```python
from build123d import *

# Parameters (mm, degrees)
SKETCH010_W     = 10
SKETCH010_H     = 20
PAD004_DEPTH    = 1.2
SKETCH011_R     = 0.7
POCKET004_DEPTH = 1.201
SKETCH012_W     = 10
SKETCH012_H     = 20
PAD005_DEPTH    = 0.2
SKETCH014_W     = 10
SKETCH014_H     = 20
PAD006_DEPTH    = 2
POCKET005_DEPTH = 2
SKETCH015_W     = 10
SKETCH015_H     = 20
PAD007_DEPTH    = 2.5
SKETCH016_R     = 2.2
SKETCH016_W     = 5.8
SKETCH016_H     = 2.7
SKETCH016_W_2   = 2.5
SKETCH016_H_2   = 10.776226
POCKET006_DEPTH = 2.5
FILLET_R        = 3


with BuildPart() as part:
    # Sketch010 → Pad004 (new body)
    with BuildSketch(Plane.XY):
        Rectangle(SKETCH010_W, SKETCH010_H)
    extrude(amount=PAD004_DEPTH)

    # Sketch011 → Pocket004 (cut, through all)
    with BuildSketch(Plane.XY.offset(1.2)):
        with Locations((-1.27, -6.75)):
            Circle(SKETCH011_R)
        with Locations((1.27, -6.75)):
            Circle(SKETCH011_R)
        with Locations((-2, 7.25)):
            Circle(SKETCH011_R)
        with Locations((-2, -1.75)):
            Circle(SKETCH011_R)
        with Locations((2, 4.02)):
            Circle(SKETCH011_R)
        with Locations((2, 1.48)):
            Circle(SKETCH011_R)
    extrude(amount=-POCKET004_DEPTH, mode=Mode.SUBTRACT)

    # Sketch012 → Pad005 (new body)
    with BuildSketch(Plane(origin=(0, 0, 0), x_dir=(1, 0, 0), z_dir=(0, 0, -1))):
        Rectangle(SKETCH012_W, SKETCH012_H)
    extrude(amount=PAD005_DEPTH)

    # Sketch014 → Pad006 (new body)
    with BuildSketch(Plane(origin=(0, 0, -0.2), x_dir=(1, 0, 0), z_dir=(0, 0, -1))):
        Rectangle(SKETCH014_W, SKETCH014_H)
    extrude(amount=PAD006_DEPTH)

    # Sketch013 → Pocket005 (cut)
    with BuildSketch(Plane(origin=(0, 0, -2.2), x_dir=(1, 0, 0), z_dir=(0, 0, -1))):
        Polygon((-3.80896, 8.420167), (3.62375, 8.420167), (3.62375, -5.103398), (0, -7.181223), (0, -8.736001), (-3.696102, -8.736001), (-3.696102, -5.976334), (0.775065, -3.412608), (0.775065, 5.283805), (-0.618984, 5.283805), (-0.618984, 0.458633), (-3.80896, 0.458633), align=None)
    extrude(amount=-POCKET005_DEPTH, mode=Mode.SUBTRACT)

    # Sketch015 → Pad007 (new body)
    with BuildSketch(Plane.XY.offset(1.2)):
        Rectangle(SKETCH015_W, SKETCH015_H)
    extrude(amount=PAD007_DEPTH)

    # Sketch016 → Pocket006 (cut)
    with BuildSketch(Plane.XY.offset(3.7)):
        with Locations((2.024904, 2.79891)):
            Circle(SKETCH016_R)
        with Locations((0, -6.75)):
            Rectangle(SKETCH016_W, SKETCH016_H)
        with Locations((-2.017145, 2.756578)):
            Rectangle(SKETCH016_W_2, SKETCH016_H_2)
    extrude(amount=-POCKET006_DEPTH, mode=Mode.SUBTRACT)

    # Fillet
    fillet_edges = [part.edges().sort_by_distance(p)[0] for p in [
        (5, -10, 0.75),
        (-5, -10, 0.75),
        (5, 10, 0.75),
        (-5, 10, 0.75),
    ]]
    fillet(fillet_edges, radius=FILLET_R)


solid = part.part
```
Geometry check sheet. Reference: the model listing, model coordinates, mm. A direction names the side the tool comes from. Round coordinates to 2 decimals unless told otherwise and drop trailing zeros. Order: outer loops, then holes, each group sorted by start corner. A loop starts at its lowest first (then second) coordinate and runs counter-clockwise, first axis right, second up. Notation, with made-up numbers: (22.5, -2) -> (29.5, -2) arc R17 cw to (29.5, 9) -> close; hole circle Ø11 at (37, -31). An arc over 180 degrees is marked (long way). Return JSON: item names as keys, results as strings. Group by question number.
Q1. Section check C-C, the plane z = 2.45. Record the boundary of the cut face in (x, y), plus the area to 3 significant figures.
Q2. Section check B-B, the plane z = -0.95. Record the boundary of the cut face in (x, y), plus the area to 3 significant figures.
Q3. Gauge pin test, flat ends, axial feed: pin 1 (1.1 mm diameter, centred on x = 1, y = -6.5, fed in from +Z); pin 2 (2 mm diameter, centred on x = -2, y = 7.25, fed in from -Z); pin 3 (0.7 mm diameter, centred on x = -2, y = 7.5, fed in from +Z). Record the tip position at first contact, or that the pin passes through.
Q4. Section check A-A, the plane y = -3.5. Record the boundary of the cut face in (x, z).
Q5. Tool access check on faces 4 (the flat face through (0, 10, 1)), 5 (the flat face through (-0.767, 3, 2)), 6 (the flat face through (0, -5.284, -1)). Record the directions out of +Z, -Z, +X, -X, +Y, -Y that give a thin tool (end or side, any length) a straight path to the whole face; none if there is none.
Q6. Release check for a two-part mould opening along X. For faces 1 (the cylindrical face through (4.1, -9.14, 0.79)), 2 (the cylindrical face through (-4.14, -9.1, 0.79)), 3 (the flat face through (-2, 8.736, -1)) record: released by +X, released by -X, zero draft, split by the parting line, or undercut.
Q7. Section check D-D, the plane z = 0.9. Record the boundary of the cut face in (x, y), plus the area to 3 significant figures.
Q8. Material ranges on probe 1 along Y at (x, z) = (-1, 1.25); probe 2 along X at (y, z) = (1.25, 2.9); probe 3 along X at (y, z) = (4.75, 2.8), recorded low to high. Write a range as from..to.
Numbers:
{
 "1": {"outline": "(-5, -7) arc R3 ccw to (-2, -10) -> (2, -10) arc R3 ccw to (5, -7) -> (5, 7) arc R3 ccw to (2, 10) -> (-2, 10) arc R3 ccw to (-5, 7) -> close; hole (-3.27, -2.63) -> (-0.77, -2.63) -> (-0.77, 8.14) -> (-3.27, 8.14) -> close; hole (-2.9, -8.1) -> (2.9, -8.1) -> (2.9, -5.4) -> (-2.9, -5.4) -> close; hole circle Ø4.4 at (2.02, 2.8)", "area": "134 mm^2"},
 "2": {"outline": "(-5, -7) arc R3 ccw to (-2, -10) -> (2, -10) arc R3 ccw to (5, -7) -> (5, 7) arc R3 ccw to (2, 10) -> (-2, 10) arc R3 ccw to (-5, 7) -> close; hole (-3.81, -8.42) -> (3.62, -8.42) -> (3.62, 5.1) -> (0, 7.18) -> (0, 8.74) -> (-3.7, 8.74) -> (-3.7, 5.98) -> (0.78, 3.41) -> (0.78, -5.28) -> (-0.62, -5.28) -> (-0.62, -0.46) -> (-3.81, -0.46) -> close", "area": "105 mm^2"},
 "3": {"pin 1": "z = 1.2", "pin 2": "z = -0.2", "pin 3": "z = 0"},
 "4": {"outline": "(-5, -2.2) -> (-3.81, -2.2) -> (-3.81, -0.2) -> (-0.62, -0.2) -> (-0.62, -2.2) -> (0.78, -2.2) -> (0.78, -0.2) -> (3.62, -0.2) -> (3.62, -2.2) -> (5, -2.2) -> (5, 3.7) -> (-5, 3.7) -> close"},
 "5": {"face 4": "+Z, -Z, +X, -X, +Y", "face 5": "+Z", "face 6": "-Z"},
 "6": {"face 1": "released by +X", "face 2": "released by -X", "face 3": "undercut"},
 "7": {"outline": "(-5, -7) arc R3 ccw to (-2, -10) -> (2, -10) arc R3 ccw to (5, -7) -> (5, 7) arc R3 ccw to (2, 10) -> (-2, 10) arc R3 ccw to (-5, 7) -> close; hole circle Ø1.4 at (-2, -1.75); hole circle Ø1.4 at (-2, 7.25); hole circle Ø1.4 at (-1.27, -6.75); hole circle Ø1.4 at (1.27, -6.75); hole circle Ø1.4 at (2, 1.48); hole circle Ø1.4 at (2, 4.02)", "area": "183 mm^2"},
 "8": {"probe 1": "-10..-8.1, -5.4..-2.63, 8.14..10", "probe 2": "-5..-3.27, -0.77..0.46, 3.59..5", "probe 3": "-5..-3.27, -0.77..1.01, 3.04..5"}
}
